Work out the finished part from the listing and answer in its coordinate system (mm). Face numbers are marked on the shaded views. A direction names the side the tool comes from. Give positions to 0.01 mm unless a question says otherwise; leave off trailing zeros. Write each loop counter-clockwise with the first axis right and the second up, starting at its lowest first coordinate (ties: lowest second). Pieces come first, ordered by that corner, then holes. Notation, with made-up numbers: (14.25, 15) -> (46.25, 15) arc R22 cw to (46.25, 47) -> close; hole circle Ø2 at (49, -27). An arc over 180 degrees is marked (long way). Write item = value, one per line. Start each with the question number.
from build123d import *

# Parameters (mm, degrees)
SKETCH_1_R               = 5.7
EXTRUDE_1_DEPTH          = 53
CUT_EXTRUDE_1_DEPTH      = 54.609514081
CUT_EXTRUDE_1_DEPTH_BACK = 54.609514081
SKETCH_2_W               = 7.04551248
SKETCH_2_H               = 6
EXTRUDE_2_DEPTH          = 10
EXTRUDE_2_DEPTH_BACK     = 10
SKETCH_2_4_W             = 7.04551248
SKETCH_2_4_H             = 6


with BuildPart() as part:
    # Sketch 1 → Extrude 1 (new body)
    with BuildSketch(Plane(origin=(0, 0, 0), x_dir=(1, 0, 0), z_dir=(0, 1, 0))):
        with Locations(Location((0, 0, 0), (0, 0, 270))):
            Circle(SKETCH_1_R)
    extrude(amount=EXTRUDE_1_DEPTH)

    # Sketch 2 → Cut-Extrude 1 (cut, two sides: drawn at the far end of the back side and taken through both)
    with BuildSketch(Plane(origin=(0, 0, 0), x_dir=(0, 0, -1), z_dir=(1, 0, 0)).offset(-CUT_EXTRUDE_1_DEPTH_BACK)):
        with Locations((0.02275624, 45.9)):
            Rectangle(SKETCH_2_W, SKETCH_2_H)
    extrude(amount=CUT_EXTRUDE_1_DEPTH + CUT_EXTRUDE_1_DEPTH_BACK, mode=Mode.SUBTRACT)

    # Sketch 2_4 → Extrude 2 (add, two sides: drawn at the far end of the back side and taken through both)
    with BuildSketch(Plane(origin=(0, 0, 0), x_dir=(0, 0, -1), z_dir=(1, 0, 0)).offset(-EXTRUDE_2_DEPTH_BACK)):
        with Locations((0.02275624, 7.1)):
            Rectangle(SKETCH_2_4_W, SKETCH_2_4_H)
    extrude(amount=EXTRUDE_2_DEPTH + EXTRUDE_2_DEPTH_BACK)


solid = part.part
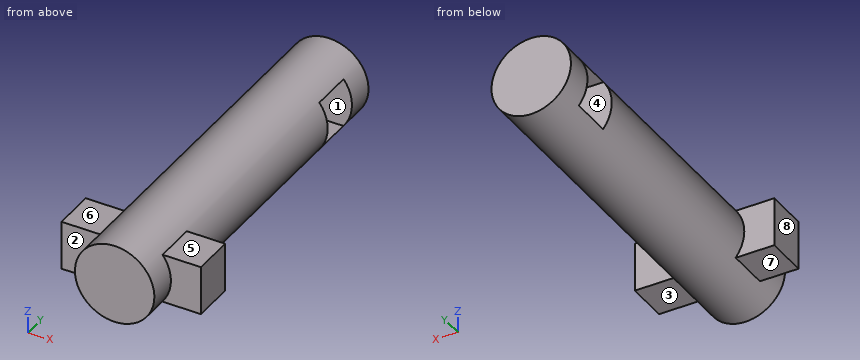
(1) A cutting plane is placed at D-D, the plane x = -2.25. Write down the section's boundary in (y, z), then the cut area to 3 significant figures.
(2) Find the intervals of material crossed by line 1 along Y through (x, z) = (-1, 0.5); line 2 along Y through (x, z) = (-9, -1.5); line 3 along X through (y, z) = (50.5, -3.5), in increasing order.
(3) A cutting plane is placed at A-A, the plane x = 0. Write down the section's boundary in (y, z), then the cut area to 3 significant figures.
(4) Each of these flat-tipped pins is pushed along its axis until it touches: pin 1 (1.5 mm diameter, centred on y = 35.5, z = -0.5, fed in from -X); pin 2 (2 mm diameter, centred on y = 47, z = 0.5, fed in from +X); pin 3 (6 mm diameter, centred on x = -8, y = 6, fed in from +Z); pin 4 (1.7 mm diameter, centred on x = -8.5, z = -0.5, fed in from +Y). Where does it stop, or does it pass through?
(5) Determine the mould class of the marked faces 1, 2, 3 and 4 for opening direction Z: pulls with the +Z half, pulls with the -Z half, needs draft (parallel to the pull), parting line crosses it, or undercut.
(6) A cutting plane is placed at B-B, the plane z = 0. Write down the section's boundary in (x, y).
(7) For the marked faces 5, 6, 7 and 8, determine the directions among +Z, -Z, +X, -X, +Y, -Y from which every point of the face is accessible in a straight line to the end or side of a thin tool.
(8) A cutting plane is placed at C-C, the plane z = 2.5. Write down the section's boundary in (x, y).
Results list:
q1.outline = (0, -5.24) -> (53, -5.24) -> (53, 5.24) -> (0, 5.24) -> close; hole (42.9, -3.55) -> (48.9, -3.55) -> (48.9, 3.5) -> (42.9, 3.5) -> close
q1.area = 513 mm²
q2.line_1 = 0 to 42.9, 48.9 to 53
q2.line_2 = 4.1 to 10.1
q2.line_3 = -4.5 to 4.5
q3.outline = (0, -5.7) -> (53, -5.7) -> (53, 5.7) -> (0, 5.7) -> close; hole (42.9, -3.55) -> (48.9, -3.55) -> (48.9, 3.5) -> (42.9, 3.5) -> close
q3.area = 562 mm²
q4.pin_1 = -5.7
q4.pin_2 = through
q4.pin_3 = 3.5
q4.pin_4 = 10.1
q5.face_1 = undercut
q5.face_2 = needs draft
q5.face_3 = pulls with the -Z half
q5.face_4 = undercut
q6.outline = (-10, 4.1) -> (-5.7, 4.1) -> (-5.7, 0) -> (5.7, 0) -> (5.7, 4.1) -> (10, 4.1) -> (10, 10.1) -> (5.7, 10.1) -> (5.7, 42.9) -> (-5.7, 42.9) -> (-5.7, 10.1) -> (-10, 10.1) -> close; (-5.7, 48.9) -> (5.7, 48.9) -> (5.7, 53) -> (-5.7, 53) -> close
q7.face_5 = +Z, +X, +Y, -Y
q7.face_6 = +Z, -X, +Y, -Y
q7.face_7 = -Z, -X, +Y, -Y
q7.face_8 = +Z, -Z, -X, +Y, -Y
q8.outline = (-10, 4.1) -> (-5.12, 4.1) -> (-5.12, 0) -> (5.12, 0) -> (5.12, 4.1) -> (10, 4.1) -> (10, 10.1) -> (5.12, 10.1) -> (5.12, 42.9) -> (-5.12, 42.9) -> (-5.12, 10.1) -> (-10, 10.1) -> close; (-5.12, 48.9) -> (5.12, 48.9) -> (5.12, 53) -> (-5.12, 53) -> close
